Could you check a few things on this drawing? It's one solid part, dimensions in mm from its lowest x, y, z. Coordinates: 2 decimals unless noted, no trailing zeros. Order: outer loops, then holes, each group sorted by start corner. A loop starts at its lowest first (then second) coordinate and runs counter-clockwise, first axis right, second up. Notation, with made-up numbers: M -20.75,19 L -7.75,19 A24 cw -7.75,55 Z; hole C 32,13 d9. An arc over 180 degrees is marked long. One line per question, with ' | ' between items. Start each with the question number.
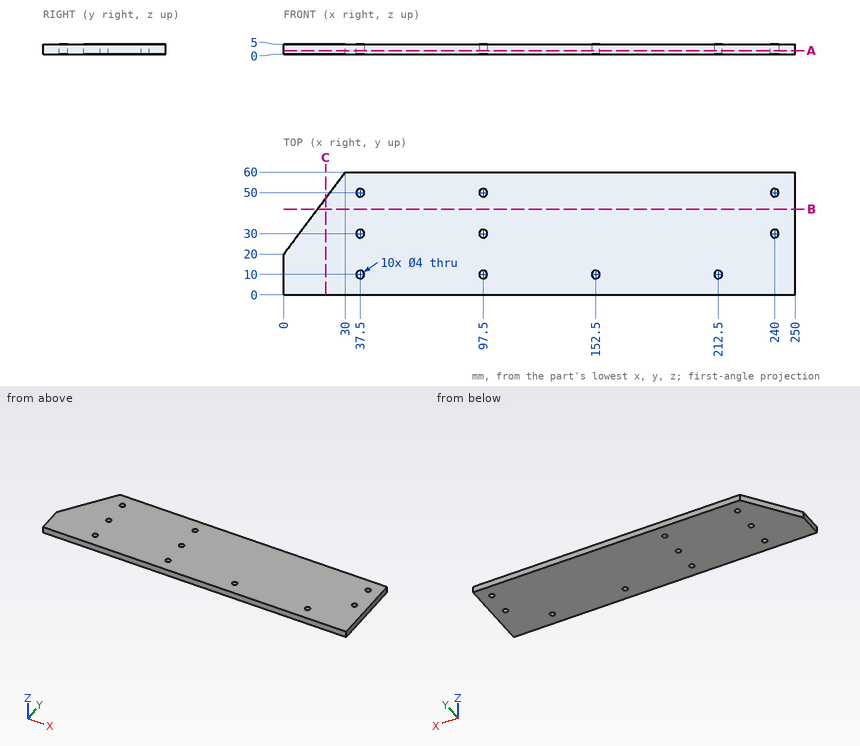
1. I need wall thicknesses on line 1 (Y direction, x = 97.5, z = 3.2); line 2 (X direction, y = 29.5, z = 1.6) (1 decimal); line 3 (Y direction, x = 212.5, z = 2.7). Which ranges of each line are inside material? Lowest first, please.
2. Will this pin go through, and if not, where does the flat tip stop? pin 1 (3.5 mm diameter, centred on x = 37.5, y = 30, fed in from -Z).
3. Imagine slicing it at B-B (y = 42). List the corners of the cut face in (x, z) for me, then the cut area to 3 significant figures.
4. Imagine slicing it at A-A (z = 1.8). Count the separate pieces of the cut face and the enclosed holes in it, then the cut area to 3 significant figures.
5. Imagine slicing it at C-C (x = 20.5). List the corners of the cut face in (y, z) for me, then the cut area to 3 significant figures.
Entries:
1) line 1: 0 to 8, 12 to 28, 32 to 48, 52 to 60 | line 2: 7.1 to 35.6, 39.4 to 95.6, 99.4 to 238.1, 241.9 to 250 | line 3: 0 to 8, 12 to 60
2) pin 1: through
3) outline: M 16.5,0 L 250,0 L 250,5 L 16.5,5 Z | area: 1,170 mm²
4) separate pieces: 1 | enclosed holes: 10 | area: 14,300 mm²
5) outline: M 0,0 L 47.33,0 L 47.33,5 L 0,5 Z | area: 237 mm²
